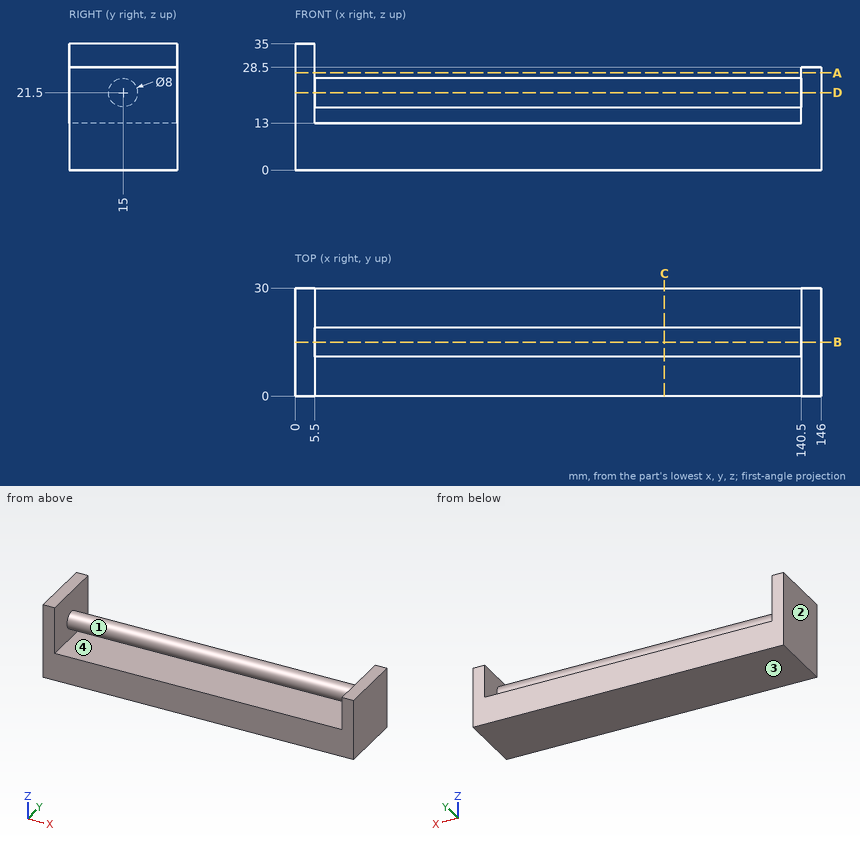
Print and shaded views of the part. All mm, measured from the part's lowest x, y and z. Coordinates: 2 decimals unless noted, no trailing zeros. Write each loop counter-clockwise with the first axis right and the second up, starting at its lowest first coordinate (ties: lowest second). Pieces come first, ordered by that corner, then holes.
(1) Cut at B-B, the plane y = 15. List the corners of the cut face in (x, z), and give its area (3 significant figures).
(2) Drill centre lines: probe 1 along X at (y, z) = (26, 15.5); probe 2 along X at (y, z) = (8.25, 30.5); probe 3 along Z at (x, y) = (83, 6.75). Where is each one in solid material? Low to high.
(3) Cut at A-A, the plane z = 27. List the corners of the cut face in (x, y).
(4) Cut at C-C, the plane x = 102.5. List the corners of the cut face in (y, z).
(5) Cut at D-D, the plane z = 21.5. List the corners of the cut face in (x, y).
(6) Flat gauge pins, fed straight in: pin 1 (8 mm diameter, centred on x = 47.5, y = 24.5, fed in from +Z); pin 2 (8 mm diameter, centred on y = 17.5, z = 20, fed in from -X); pin 3 (4 mm diameter, centred on x = 56, y = 17.5, fed in from +Z); pin 4 (5 mm diameter, centred on x = 83, z = 25.5, fed in from -Y). Where does each tip first touch, or does it go through?
(7) Two-plate mould, pull along Z, no slides. Class the marked faces 1, 2, 3 and 4: +Z half, -Z half, draft (parallel to the pull), parting line (faces both ways), or undercut.
Geometry says:
1. outline: (0, 0) - (146, 0) - (146, 28.5) - (140.5, 28.5) - (140.5, 25.5) - (5.5, 25.5) - (5.5, 35) - (0, 35) - close; hole (5.5, 13) - (140.5, 13) - (140.5, 17.5) - (5.5, 17.5) - close
1. area: 3,180 mm2
2. probe 1: x = 0 to 5.5, 140.5 to 146
2. probe 2: x = 0 to 5.5
2. probe 3: z = 0 to 13
3. outline: (0, 0) - (5.5, 0) - (5.5, 30) - (0, 30) - close; (140.5, 0) - (146, 0) - (146, 30) - (140.5, 30) - close
4. outline: (0, 0) - (30, 0) - (30, 13) - (0, 13) - close; circle Ø8 at (15, 21.5)
5. outline: (0, 0) - (5.5, 0) - (5.5, 11) - (140.5, 11) - (140.5, 0) - (146, 0) - (146, 30) - (140.5, 30) - (140.5, 19) - (5.5, 19) - (5.5, 30) - (0, 30) - close
6. pin 1: stops at z = 13
6. pin 2: stops at x = 0
6. pin 3: stops at z = 25.47
6. pin 4: stops at y = 11.29
7. face 1: undercut
7. face 2: draft
7. face 3: -Z half
7. face 4: undercut
